Can you work these out from the model? Positions are in its coordinate system, mm. A direction names the side the tool comes from. Round coordinates to 2 decimals unless told otherwise and drop trailing zeros. Write each loop counter-clockwise with the first axis right and the second up, starting at its lowest first coordinate (ties: lowest second). Pieces come first, ordered by that corner, then holes.
Q1. If we section it at D-D (y = 33.5): Please give me the cut outline in (x, z), plus the area to 3 significant figures.
Q2. I'm going to push flat-ended pins straight in: pin 1 Ø1.5 at (x, z) = (12, 0.5) entering from +Y; pin 2 Ø2 at (x, z) = (10, 1.5) entering from +Y; pin 3 Ø2.5 at (x, z) = (11, 0) entering from -Y; pin 4 Ø8 at (x, y) = (7, 33) entering from -Z. Where does each tip first touch, or does it pass through?
Q3. We'd pull the mould along Y, two halves only. Please class faces 1 (the flat face through (7, 25, 6.5)), 2 (the cylindrical face through (11.77, 34.5, -9.46)), 3 (the cylindrical face through (6.9, 11.5, -5.07)): +Y half, -Y half, draft (parallel to the pull), parting line (faces both ways), or undercut.
Q4. Please list where these lines run through material, in increasing order: line 1 along Y through (x, z) = (7, 7.7); line 2 along Z through (x, y) = (11.5, 15); line 3 along X through (y, z) = (30, -10.5).
Q5. If we section it at A-A (y = 11): Please give me the cut outline in (x, z).
Q6. For faces 4 (the flat face through (7, 15, -12.5)), 5 (the flat face through (1, 10, 0)), 6 (the cylindrical face through (11.77, 34.5, 9.04)), which set-ups out of +Z, -Z, +X, -X, +Y, -Y let a thin tool reach every point of the face, with its end or its side?
Q7. If we section it at B-B (z = 0): Please give me the cut outline in (x, y), plus the area to 3 significant figures.
Q8. If we section it at C-C (x = 6.25): Please give me the cut outline in (y, z), plus the area to 3 significant figures.
from build123d import *

# Parameters (mm, degrees)
EXTRUDE_1_DEPTH     = 14
FILLET_1_R          = 7
CUT_EXTRUDE_START   = -1
SKETCH_7_R          = 5
CUT_EXTRUDE_1_DEPTH = 31
SKETCH_8_R          = 3.1
CUT_EXTRUDE_2_DEPTH = 35
SKETCH_10_R         = 1.5
CUT_EXTRUDE_3_DEPTH = 20


with BuildPart() as part:
    # 草图4 → 凸台-拉伸1 (new body)
    with BuildSketch(Plane(origin=(0, 0, 0), x_dir=(0, 0, -1), z_dir=(1, 0, 0))):
        with BuildLine():
            Line((0, 0), (12.5, 0))
            Line((12.5, 0), (12.5, 40))
            Line((12.5, 40), (6.5, 40))
            Line((6.5, 40), (6.5, 15))
            ThreePointArc((6.5, 15), (5.035533906, 11.464466094), (1.5, 10))
            Line((1.5, 10), (-1.5, 10))
            ThreePointArc((-1.5, 10), (-5.035533906, 11.464466094), (-6.5, 15))
            Line((-6.5, 15), (-6.5, 40))
            Line((-6.5, 40), (-12.5, 40))
            Line((-12.5, 40), (-12.5, 0))
            Line((-12.5, 0), (0, 0))
        make_face()
    extrude(amount=EXTRUDE_1_DEPTH)

    # 圆角1
    fillet_1_edges = [part.edges().sort_by_distance(p)[0] for p in [
        (0, 40, 9.5),
        (0, 40, -9.5),
        (14, 40, -9.5),
        (14, 40, 9.5),
    ]]
    fillet(fillet_1_edges, radius=FILLET_1_R - 0.0001)  # a hair under: the kernel refuses the full size

    # 草图7 → 切除-拉伸1 (cut)
    with BuildSketch(Plane.XY.offset(12.5).offset(CUT_EXTRUDE_START)):
        with Locations((7, 33)):
            Circle(SKETCH_7_R)
    extrude(amount=-CUT_EXTRUDE_1_DEPTH, mode=Mode.SUBTRACT)

    # 草图8 → 切除-拉伸2 (cut)
    with BuildSketch(Plane.XY.offset(12.5)):
        with Locations((7, 33)):
            Circle(SKETCH_8_R)
    extrude(amount=-CUT_EXTRUDE_2_DEPTH, mode=Mode.SUBTRACT)

    # 草图10 → 切除-拉伸3 (cut)
    with BuildSketch(Plane(origin=(0, 10, 0), x_dir=(1, 0, 0), z_dir=(0, 1, 0))):
        with Locations(Location((3, 0, 0), (0, 0, 270))):
            Circle(SKETCH_10_R)
        with Locations(Location((11, 0, 0), (0, 0, 270))):
            Circle(SKETCH_10_R)
    extrude(amount=-CUT_EXTRUDE_3_DEPTH, mode=Mode.SUBTRACT)


solid = part.part
A:
1. outline: (0.02, -12.5) - (2.03, -12.5) - (2.03, -6.5) - (0.02, -6.5) - close; (0.02, 6.5) - (2.03, 6.5) - (2.03, 11.5) - (3.94, 11.5) - (3.94, 12.5) - (0.02, 12.5) - close; (10.06, 11.5) - (11.97, 11.5) - (11.97, 6.5) - (13.98, 6.5) - (13.98, 12.5) - (10.06, 12.5) - close; (11.97, -12.5) - (13.98, -12.5) - (13.98, -6.5) - (11.97, -6.5) - close
1. area: 52.0 mm2
2. pin 1: stops at y = 10
2. pin 2: stops at y = 10.1
2. pin 3: passes through
2. pin 4: stops at z = 11.5
3. face 1: draft
3. face 2: undercut
3. face 3: +Y half
4. line 1: y = 0 to 28, 38 to 40
4. line 2: z = -12.5 to -6.5, 6.5 to 12.5
4. line 3: x = 0 to 3, 11 to 14
5. outline: (0, -12.5) - (14, -12.5) - (14, -4.5) - (0, -4.5) - close; (0, 4.5) - (14, 4.5) - (14, 12.5) - (0, 12.5) - close
6. face 4: -Z, +X, -X, +Y, -Y
6. face 5: +X, -X, +Y
6. face 6: -Z
7. outline: (0, 0) - (1.5, 0) - (1.5, 10) - (0, 10) - close; (4.5, 0) - (9.5, 0) - (9.5, 10) - (4.5, 10) - close; (12.5, 0) - (14, 0) - (14, 10) - (12.5, 10) - close
7. area: 80.0 mm2
8. outline: (0, -12.5) - (28.06, -12.5) - (28.06, -6.5) - (15, -6.5) arc R5 cw to (10, -1.5) - (10, 1.5) arc R5 cw to (15, 6.5) - (28.06, 6.5) - (28.06, 11.5) - (29.99, 11.5) - (29.99, 12.5) - (0, 12.5) - close; (36.01, 11.5) - (37.94, 11.5) - (37.94, 6.5) - (39.96, 6.5) - (39.96, 12.5) - (36.01, 12.5) - close; (37.94, -12.5) - (39.96, -12.5) - (39.96, -6.5) - (37.94, -6.5) - close
8. area: 505 mm2
